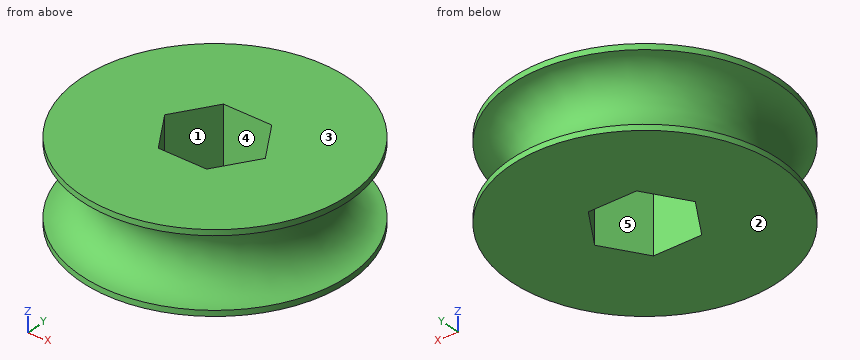
from build123d import *

# Parameters (mm, degrees)
SKETCH1_R           = 50
BOSS_EXTRUDE1_DEPTH = 30
SKETCH2_R           = 12.893523165


with BuildPart() as part:
    # Sketch1 → Boss-Extrude1 (new body)
    with BuildSketch(Plane.XY):
        Circle(SKETCH1_R)
        Polygon((-9, 15.15359655), (9, 15.15359655), (18.714345659, 0), (9, -15.15359655), (-9, -15.15359655), (-18.714345659, 0), align=None, mode=Mode.SUBTRACT)
    extrude(amount=BOSS_EXTRUDE1_DEPTH)

    # Sketch2 → Cut-Revolve1 (revolve, cut)
    with BuildSketch(Plane(origin=(0, 0, 0), x_dir=(0, 0, -1), z_dir=(1, 0, 0)), mode=Mode.PRIVATE) as cut_revolve1_sk:
        with Locations((-15, 50)):
            Circle(SKETCH2_R)
    revolve(cut_revolve1_sk.sketch.rotate(Axis((0, 0, -15.913585238), (0, 0, 1)), 90), axis=Axis((0, 0, -15.913585238), (0, 0, 1)), mode=Mode.SUBTRACT)


solid = part.part
Verification items for the finished model (mm, model axes). Face numbers are marked on the shaded views. A direction names the side the tool comes from. Round coordinates to 2 decimals unless told otherwise and drop trailing zeros. Loops run counter-clockwise (first coordinate to the right, second up) from the corner with the lowest first, then second, coordinate; pieces in that order, holes last. Notation, with made-up numbers: (75.25, 56.5) - (85.25, 56.5) arc R28 cw to (85.25, 78.5) - close; hole circle Ø4 at (88, 21.5). An arc over 180 degrees is marked (long way). Use one line per item in the form item = value.
1. Section check B-B on z = 8.5. Record the cut outline in (x, y).
A:
outline = circle Ø77.73 at (0, 0); hole (-18.71, 0) - (-9, -15.15) - (9, -15.15) - (18.71, 0) - (9, 15.15) - (-9, 15.15) - close
2. Section check A-A on x = 0. Record the cut outline in (y, z).
A:
outline = (-50, 0) - (-15.15, 0) - (-15.15, 30) - (-50, 30) - (-50, 27.89) arc R12.89 cw to (-50, 2.11) - close; (15.15, 0) - (50, 0) - (50, 2.11) arc R12.89 cw to (50, 27.89) - (50, 30) - (15.15, 30) - close
3. Gauge pin test, flat ends, axial feed: pin 1 Ø8 at (x, z) = (6.5, 13) entering from -Y; pin 2 Ø2 at (x, z) = (-29, 25) entering from -Y; pin 3 Ø1.5 at (x, z) = (-20, 6.5) entering from +Y; pin 4 Ø4 at (x, y) = (35, -29) entering from -Z. Record the tip position at first contact, or that the pin passes through.
A:
pin_1 = -38.13
pin_2 = -32.3
pin_3 = 35.9
pin_4 = 0
4. Draft check along Y on the marked faces 3, 4 and 5. Enter one of: pulls with the +Y half, pulls with the -Y half, needs draft (parallel to the pull), parting line crosses it, or undercut.
A:
face_3 = needs draft
face_4 = undercut
face_5 = undercut
5. Scan lines: probe 1 along Z at (x, y) = (45, -20); probe 2 along Z at (x, y) = (-18.5, -41.5); probe 3 along Y at (x, z) = (17, 12.5). Record each from-to range of solid material in increasing order.
A:
probe_1 = 0 to 2.13, 27.87 to 30
probe_2 = 0 to 2.94, 27.06 to 30
probe_3 = -33.26 to -2.67, 2.67 to 33.26
6. Access from +Z, -Z, +X, -X, +Y, -Y to the whole of each face (thin tool, end or side, straight path). Record for the marked faces 1 and 2.
A:
face_1 = +Z, -Z
face_2 = -Z, +X, -X, +Y, -Y
7. Section check C-C on z = 18.5. Record the cut outline in (x, y).
A:
outline = circle Ø75.18 at (0, 0); hole (-18.71, 0) - (-9, -15.15) - (9, -15.15) - (18.71, 0) - (9, 15.15) - (-9, 15.15) - close
